from build123d import *

# Parameters (mm, degrees)
SKETCH1_R           = 34.925
BOSS_EXTRUDE1_DEPTH = 4.7625


with BuildPart() as part:
    # Sketch1 → Boss-Extrude1 (new body)
    with BuildSketch(Plane.XY):
        Circle(SKETCH1_R)
        with BuildLine():
            ThreePointArc((2.243888697, 8.727933453), (-0.797066547, 7.281111303), (-2.243888697, 10.322066547))
            ThreePointArc((-2.243888697, 10.322066547), (9.70011878, 20.108105734), (23.923949148, 14.099068603))
            ThreePointArc((23.923949148, 14.099068603), (23.396113859, 10.773096108), (20.070141364, 11.300931397))
            ThreePointArc((20.070141364, 11.300931397), (10.380475923, 15.394453179), (2.243888697, 8.727933453))
        make_face(mode=Mode.SUBTRACT)
        with BuildLine():
            ThreePointArc((5.712134337, 8.885472165), (21.077597689, 7.359558154), (26.886333692, -6.947239658))
            ThreePointArc((26.886333692, -6.947239658), (24.161280075, -8.92582145), (22.182698283, -6.200767833))
            ThreePointArc((22.182698283, -6.200767833), (18.225627153, 3.545417318), (7.758249844, 4.584912017))
            ThreePointArc((7.758249844, 4.584912017), (4.584912017, 5.712134337), (5.712134337, 8.885472165))
        make_face(mode=Mode.SUBTRACT)
        with BuildLine():
            ThreePointArc((10.322066547, 2.243888697), (20.108105734, -9.70011878), (14.099068603, -23.923949148))
            ThreePointArc((14.099068603, -23.923949148), (10.773096108, -23.396113859), (11.300931397, -20.070141364))
            ThreePointArc((11.300931397, -20.070141364), (15.394453179, -10.380475923), (8.727933453, -2.243888697))
            ThreePointArc((8.727933453, -2.243888697), (7.281111303, 0.797066547), (10.322066547, 2.243888697))
        make_face(mode=Mode.SUBTRACT)
        with BuildLine():
            ThreePointArc((8.885472165, -5.712134337), (7.359558154, -21.077597689), (-6.947239658, -26.886333692))
            ThreePointArc((-6.947239658, -26.886333692), (-8.92582145, -24.161280075), (-6.200767833, -22.182698283))
            ThreePointArc((-6.200767833, -22.182698283), (3.545417318, -18.225627153), (4.584912017, -7.758249844))
            ThreePointArc((4.584912017, -7.758249844), (5.712134337, -4.584912017), (8.885472165, -5.712134337))
        make_face(mode=Mode.SUBTRACT)
        with BuildLine():
            ThreePointArc((2.243888697, -10.322066547), (-9.70011878, -20.108105734), (-23.923949148, -14.099068603))
            ThreePointArc((-23.923949148, -14.099068603), (-23.396113859, -10.773096108), (-20.070141364, -11.300931397))
            ThreePointArc((-20.070141364, -11.300931397), (-10.380475923, -15.394453179), (-2.243888697, -8.727933453))
            ThreePointArc((-2.243888697, -8.727933453), (0.797066547, -7.281111303), (2.243888697, -10.322066547))
        make_face(mode=Mode.SUBTRACT)
        with BuildLine():
            ThreePointArc((-5.712134337, -8.885472165), (-21.077597689, -7.359558154), (-26.886333692, 6.947239658))
            ThreePointArc((-26.886333692, 6.947239658), (-24.161280075, 8.92582145), (-22.182698283, 6.200767833))
            ThreePointArc((-22.182698283, 6.200767833), (-18.225627153, -3.545417318), (-7.758249844, -4.584912017))
            ThreePointArc((-7.758249844, -4.584912017), (-4.584912017, -5.712134337), (-5.712134337, -8.885472165))
        make_face(mode=Mode.SUBTRACT)
        with BuildLine():
            ThreePointArc((-10.322066547, -2.243888697), (-20.108105734, 9.70011878), (-14.099068603, 23.923949148))
            ThreePointArc((-14.099068603, 23.923949148), (-10.773096108, 23.396113859), (-11.300931397, 20.070141364))
            ThreePointArc((-11.300931397, 20.070141364), (-15.394453179, 10.380475923), (-8.727933453, 2.243888697))
            ThreePointArc((-8.727933453, 2.243888697), (-7.281111303, -0.797066547), (-10.322066547, -2.243888697))
        make_face(mode=Mode.SUBTRACT)
        with BuildLine():
            ThreePointArc((-8.885472165, 5.712134337), (-7.359558154, 21.077597689), (6.947239658, 26.886333692))
            ThreePointArc((6.947239658, 26.886333692), (8.92582145, 24.161280075), (6.200767833, 22.182698283))
            ThreePointArc((6.200767833, 22.182698283), (-3.545417318, 18.225627153), (-4.584912017, 7.758249844))
            ThreePointArc((-4.584912017, 7.758249844), (-5.712134337, 4.584912017), (-8.885472165, 5.712134337))
        make_face(mode=Mode.SUBTRACT)
    extrude(amount=BOSS_EXTRUDE1_DEPTH)


solid = part.part
Model file for the job. Use its own axes, mm. A direction names the side the tool comes from. Give positions to 0.01 mm unless a question says otherwise; leave off trailing zeros. Order: outer loops, then holes, each group sorted by start corner. A loop starts at its lowest first (then second) coordinate and runs counter-clockwise, first axis right, second up. Notation, with made-up numbers: (22, -3.5) - (41, -3.5) arc R27 ccw to (41, 24.5) - close; hole circle Ø2 at (-18.75, -2). An arc over 180 degrees is marked (long way). Return JSON: item names as keys, results as strings.
1) Probe line 1 (Y direction, x = -13, z = 1.25); line 2 (Y direction, x = 12, z = 2.9); line 3 (X direction, y = -13, z = 3.4). List the from-to ranges inside material, lowest first. Write a range as from..to.
Geometry says:
{"line 1": "-32.42..-20.22, -15.43..-10.31, -5.53..-0.98, 5.15..18.51, 24.36..32.42", "line 2": "-32.8..-24.27, -19.51..-4.15, 1.53..5.57, 10.33..15.5, 20.26..32.8", "line 3": "-32.42..-24.36, -18.51..-5.15, 0.98..5.53, 10.31..15.43, 20.22..32.42"}
2) Cut at C-C, the plane z = 2.55. Count the separate pieces of the cut face and the enclosed holes in it, plus the area to 3 significant figures.
Geometry says:
{"separate pieces": "1", "enclosed holes": "8", "area": "2,650 mm²"}
3) Pull direction Y, two halves, no side cores. Call faces 1 (the cylindrical face through (4.608, 5.665, 2.348)), 2 (the cylindrical face through (-27.715, -21.251, 2.348)), 3 (the flat face through (0, 0, 4.762)): pulls with the +Y half, pulls with the -Y half, needs draft (parallel to the pull), parting line crosses it, or undercut.
Geometry says:
{"face 1": "undercut", "face 2": "parting line crosses it", "face 3": "needs draft"}
4) Flat gauge pins, fed straight in: P1, Ø1.5, axis at x = 7.5, z = 1.5, coming from the +Y side; P2, Ø2, axis at y = -21.5, z = 3.5, coming from the -X side; P3, Ø2, axis at y = -13, z = 0.5, coming from the +X side. Where does each tip first touch, or does it go through?
Geometry says:
{"P1": "y = 34.27", "P2": "x = -28.28", "P3": "x = 32.8"}
5) 3-axis set-ups, long thin cutter, end or side, ignore diameter. For faces 4 (the flat face through (0, 0, 0)), 5 (the cylindrical face through (-10.534, -15.415, 2.348)): which of +Z, -Z, +X, -X, +Y, -Y reach the whole face in a straight line?
Geometry says:
{"face 4": "-Z, +X, -X, +Y, -Y", "face 5": "+Z, -Z"}
6) Cut at A-A, the plane y = 12.7. Give the cut face in (x, z), plus the area to 3 significant figures.
Geometry says:
{"outline": "(-32.53, 0) - (-20.24, 0) - (-20.24, 4.76) - (-32.53, 4.76) - close; (-15.46, 0) - (-10.32, 0) - (-10.32, 4.76) - (-15.46, 4.76) - close; (-5.56, 0) - (-1.16, 0) - (-1.16, 4.76) - (-5.56, 4.76) - close; (4.82, 0) - (18.84, 0) - (18.84, 4.76) - (4.82, 4.76) - close; (24.38, 0) - (32.53, 0) - (32.53, 4.76) - (24.38, 4.76) - close", "area": "210 mm²"}
